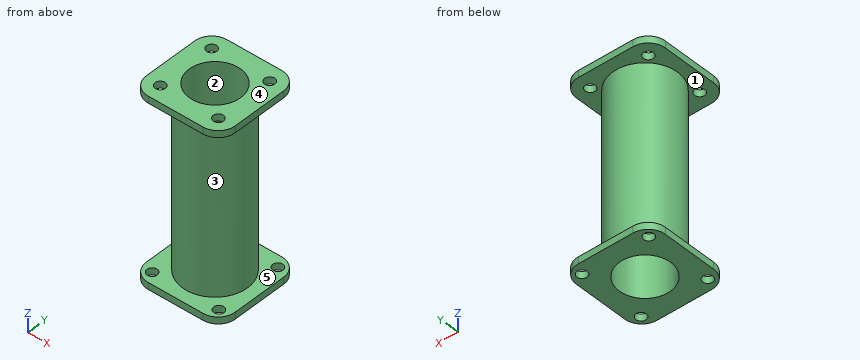
from build123d import *

# Parameters (mm, degrees)
SKETCH_1_R      = 9.5
SKETCH_1_R_2    = 1.5
EXTRUDE_1_DEPTH = 2
SKETCH_1_6_R    = 9.5
SKETCH_1_6_R_2  = 7.5
EXTRUDE_2_DEPTH = 55
EXTRUDE_START   = -2
SKETCH_5_R      = 1.5
SKETCH_5_R_2    = 9.5
EXTRUDE_3_DEPTH = 2


with BuildPart() as part:
    # Sketch 1 → Extrude 1 (new body)
    with BuildSketch(Plane.XY):
        with BuildLine():
            Line((-8, 13), (8, 13))
            ThreePointArc((8, 13), (11.535533906, 11.535533906), (13, 8))
            Line((13, 8), (13, -8))
            ThreePointArc((13, -8), (11.535533906, -11.535533906), (8, -13))
            Line((8, -13), (-8, -13))
            ThreePointArc((-8, -13), (-11.535533906, -11.535533906), (-13, -8))
            Line((-13, -8), (-13, 8))
            ThreePointArc((-13, 8), (-11.535533906, 11.535533906), (-8, 13))
        make_face()
        Circle(SKETCH_1_R, mode=Mode.SUBTRACT)
        with Locations((-9.767766953, 9.767766953)):
            Circle(SKETCH_1_R_2, mode=Mode.SUBTRACT)
        with Locations((-9.767766953, -9.767766953)):
            Circle(SKETCH_1_R_2, mode=Mode.SUBTRACT)
        with Locations((9.767766953, 9.767766953)):
            Circle(SKETCH_1_R_2, mode=Mode.SUBTRACT)
        with Locations((9.767766953, -9.767766953)):
            Circle(SKETCH_1_R_2, mode=Mode.SUBTRACT)
    extrude(amount=EXTRUDE_1_DEPTH)

    # Sketch 1_6 → Extrude 2 (add)
    with BuildSketch(Plane.XY):
        Circle(SKETCH_1_6_R)
        Circle(SKETCH_1_6_R_2, mode=Mode.SUBTRACT)
    extrude(amount=EXTRUDE_2_DEPTH)

    # Sketch 5 → Extrude 3 (add)
    with BuildSketch(Plane.XY.offset(55).offset(EXTRUDE_START)):
        with BuildLine():
            Line((8, 13), (-8, 13))
            ThreePointArc((-8, 13), (-11.535533906, 11.535533906), (-13, 8))
            Line((-13, 8), (-13, -8))
            ThreePointArc((-13, -8), (-11.535533906, -11.535533906), (-8, -13))
            Line((-8, -13), (8, -13))
            ThreePointArc((8, -13), (11.535533906, -11.535533906), (13, -8))
            Line((13, -8), (13, 8))
            ThreePointArc((13, 8), (11.535533906, 11.535533906), (8, 13))
        make_face()
        with Locations((-8.5, -8.5)):
            Circle(SKETCH_5_R, mode=Mode.SUBTRACT)
        with Locations((8.5, -8.5)):
            Circle(SKETCH_5_R, mode=Mode.SUBTRACT)
        Circle(SKETCH_5_R_2, mode=Mode.SUBTRACT)
        with Locations((-8.5, 8.5)):
            Circle(SKETCH_5_R, mode=Mode.SUBTRACT)
        with Locations((8.5, 8.5)):
            Circle(SKETCH_5_R, mode=Mode.SUBTRACT)
    extrude(amount=EXTRUDE_3_DEPTH)


solid = part.part
Part model, mm, in its own coordinate system. Face numbers are marked on the shaded views. A direction names the side the tool comes from. Give positions to 0.01 mm unless a question says otherwise; leave off trailing zeros. Order: outer loops, then holes, each group sorted by start corner. A loop starts at its lowest first (then second) coordinate and runs counter-clockwise, first axis right, second up. Notation, with made-up numbers: (-24, -12.75) -> (3, -12.75) arc R23 cw to (3, 19.25) -> close; hole circle Ø7 at (73.5, -36.5). An arc over 180 degrees is marked (long way). Use one line per item in the form item = value.
(1) Saw through at A-A (x = 0). Write the cut outline in (y, z).
Solution:
outline = (-13, 0) -> (-7.5, 0) -> (-7.5, 55) -> (-13, 55) -> (-13, 53) -> (-9.5, 53) -> (-9.5, 2) -> (-13, 2) -> close; (7.5, 0) -> (13, 0) -> (13, 2) -> (9.5, 2) -> (9.5, 53) -> (13, 53) -> (13, 55) -> (7.5, 55) -> close
(2) Drill centre lines: line 1 (Z direction, x = -3, y = 9.5); line 2 (Y direction, x = 0, z = 20); line 3 (Y direction, x = 8.5, z = 54.25). Where is each one in solid material? Low to high. Write a range as from..to.
Solution:
line_1 = 0..2, 53..55
line_2 = -9.5..-7.5, 7.5..9.5
line_3 = -12.97..-10, -7..7, 10..12.97
(3) Tool access for the marked faces 4 and 5: list every direction of +Z, -Z, +X, -X, +Y, -Y with a clear straight run to the whole face (end or side of a thin tool).
Solution:
face_4 = +Z, +X, -X, +Y, -Y
face_5 = none
(4) Saw through at C-C (z = 20). Write the cut outline in (x, y), then the cut area to 3 significant figures.
Solution:
outline = circle Ø19 at (0, 0); hole circle Ø15 at (0, 0)
area = 107 mm²
(5) Flat gauge pins, fed straight in: P1, Ø2.5, axis at x = -8.5, y = 8.5, coming from the +Z side; P2, Ø1.5, axis at y = 4, z = 11, coming from the +X side; P3, Ø4, axis at y = 3.5, z = 48.5, coming from the -X side; P4, Ø13.5, axis at x = 0, y = 0, coming from the -Z side. Where does each tip first touch, or does it go through?
Solution:
P1 = 2
P2 = 8.93
P3 = -9.38
P4 = through
(6) Pull direction Y, two halves, no side cores. Call the marked faces 1, 2 and 3: +Y half, -Y half, draft (parallel to the pull), parting line (faces both ways), or undercut.
Solution:
face_1 = draft
face_2 = undercut
face_3 = parting line
(7) Saw through at B-B (y = 3.5). Write the cut outline in (x, z), then the cut area to 3 significant figures.
Solution:
outline = (-13, 0) -> (-6.63, 0) -> (-6.63, 55) -> (-13, 55) -> (-13, 53) -> (-8.83, 53) -> (-8.83, 2) -> (-13, 2) -> close; (6.63, 0) -> (13, 0) -> (13, 2) -> (8.83, 2) -> (8.83, 53) -> (13, 53) -> (13, 55) -> (6.63, 55) -> close
area = 275 mm²
